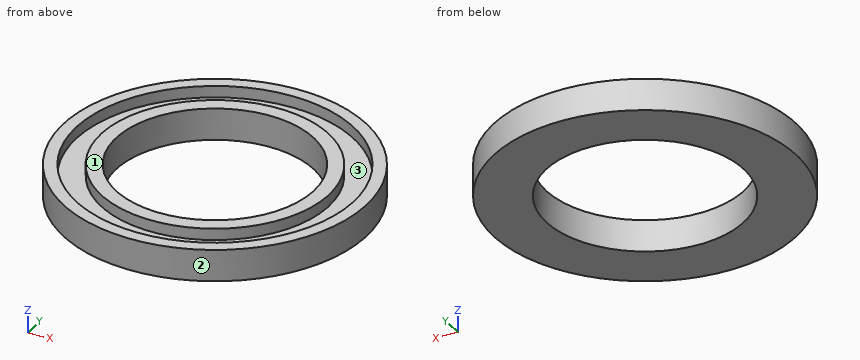
```python
from build123d import *

# Parameters (mm, degrees)
SKETCH_R      = 26.2
SKETCH_R_2    = 17.1
PAD_DEPTH     = 5.5
SKETCH001_R   = 24
SKETCH001_R_2 = 19.7
POCKET_DEPTH  = 2


with BuildPart() as part:
    # Sketch → Pad (new body)
    with BuildSketch(Plane.XY):
        Circle(SKETCH_R)
        Circle(SKETCH_R_2, mode=Mode.SUBTRACT)
    extrude(amount=PAD_DEPTH)

    # Sketch001 → Pocket (cut)
    with BuildSketch(Plane.XY.offset(5.5)):
        Circle(SKETCH001_R)
        Circle(SKETCH001_R_2, mode=Mode.SUBTRACT)
    extrude(amount=-POCKET_DEPTH, mode=Mode.SUBTRACT)


solid = part.part
```
Geometry: final body of the model. Coordinates: model frame, mm. Face numbers are marked on the shaded views. Round coordinates to 2 decimals unless told otherwise and drop trailing zeros. Write each loop counter-clockwise with the first axis right and the second up, starting at its lowest first coordinate (ties: lowest second). Pieces come first, ordered by that corner, then holes.
Item 1: Section query D-D (y = -20.5). Return loops of the section in (x, z).
Item 2: Material intervals for L1, parallel to Y at x = 0, z = 3.95; L2, parallel to Y at x = 0, z = 1.5; L3, parallel to X at y = 5.5, z = 4.4, sorted ascending.
Item 3: Pin query (flat end, axial travel): P1, Ø12, axis at x = 8, y = 3.5, coming from the +Z side. Return the tip coordinate at first contact, or that it passes through.
Item 4: Section query A-A (x = 0). Return loops of the section in (y, z).
Item 5: Mould query, pull axis Y, two halves, no side actions, for the marked faces 1, 2 and 3. Classes: +Y half, -Y half, draft (parallel to the pull), parting line (faces both ways), or undercut.
Item 6: Section query C-C (z = 4.55). Return loops of the section in (x, y).
Completed:
1. outline: (-16.32, 0) - (16.32, 0) - (16.32, 5.5) - (12.48, 5.5) - (12.48, 3.5) - (-12.48, 3.5) - (-12.48, 5.5) - (-16.32, 5.5) - close
2. L1: y = -26.2 to -24, -19.7 to -17.1, 17.1 to 19.7, 24 to 26.2
2. L2: y = -26.2 to -17.1, 17.1 to 26.2
2. L3: x = -25.62 to -23.36, -18.92 to -16.19, 16.19 to 18.92, 23.36 to 25.62
3. P1: passes through
4. outline: (-26.2, 0) - (-17.1, 0) - (-17.1, 5.5) - (-19.7, 5.5) - (-19.7, 3.5) - (-24, 3.5) - (-24, 5.5) - (-26.2, 5.5) - close; (17.1, 0) - (26.2, 0) - (26.2, 5.5) - (24, 5.5) - (24, 3.5) - (19.7, 3.5) - (19.7, 5.5) - (17.1, 5.5) - close
5. face 1: draft
5. face 2: parting line
5. face 3: undercut
6. outline: circle Ø52.4 at (0, 0); circle Ø39.4 at (0, 0); hole circle Ø48 at (0, 0); hole circle Ø34.2 at (0, 0)
